from build123d import *

# Parameters (mm, degrees)
F0_R     = 19.05
F0_R_2   = 6.35
F1_DEPTH = 50.8
F3_DEPTH = 12.7


with BuildPart() as f1:
    # F0 (on Front) → F1 (new body, symmetric)
    with BuildSketch(Plane.XZ):
        Circle(F0_R)
        Circle(F0_R_2, mode=Mode.SUBTRACT)
    extrude(amount=F1_DEPTH, both=True)

    # F2 (on face) → F3 (join)
    with BuildSketch(Plane.XZ.offset(50.8)):
        with BuildLine():
            Line((-19.05, 50.8), (-19.05, 0))
            ThreePointArc((-19.05, 0), (0, 19.05), (19.05, 0))
            Line((19.05, 0), (19.05, 50.8))
            ThreePointArc((19.05, 50.8), (0, 31.75), (-19.05, 50.8))
        make_face()
        with BuildLine():
            ThreePointArc((19.05, 50.8), (0, 69.85), (-19.05, 50.8))
            Line((-19.05, 50.8), (-6.35, 50.8))
            ThreePointArc((-6.35, 50.8), (0, 57.15), (6.35, 50.8))
            Line((6.35, 50.8), (19.05, 50.8))
        make_face()
        with BuildLine():
            Line((-6.35, 50.8), (-19.05, 50.8))
            ThreePointArc((-19.05, 50.8), (0, 31.75), (19.05, 50.8))
            Line((19.05, 50.8), (6.35, 50.8))
            ThreePointArc((6.35, 50.8), (0, 44.45), (-6.35, 50.8))
        make_face()
    extrude(amount=-F3_DEPTH)

    # F4: F1 across plane


with BuildPart() as f1_1:
    add(f1.part)
    add(f1.part.mirror(Plane.XZ))


solid = f1_1.part
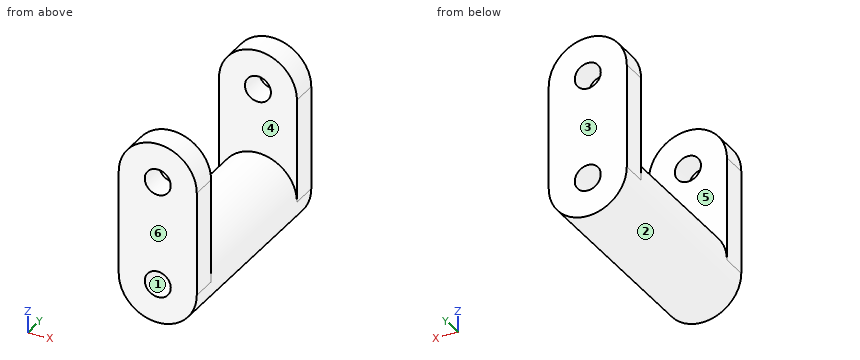
For this review, take the finished solid that the model builds, in its own axes (mm). Face numbers are marked on the shaded views. A direction names the side the tool comes from. Round coordinates to 2 decimals unless told otherwise and drop trailing zeros. Order: outer loops, then holes, each group sorted by start corner. A loop starts at its lowest first (then second) coordinate and runs counter-clockwise, first axis right, second up. Notation, with made-up numbers: M -26.5,-30.5 L -12.5,-30.5 A19 ccw -12.5,3.5 Z; hole C -29,-9.5 d5. An arc over 180 degrees is marked long. Write each question's results on one line, items separated by ' | '. Start each with the question number.
1. Draft analysis for pull direction Y (two halves, no side actions). For the marked faces 3, 4, 5 and 6, state which applies: pulls with the +Y half, pulls with the -Y half, needs draft (parallel to the pull), parting line crosses it, or undercut.
2. Add section C-C (y = -27.5). State the section outline as (x, z) points.
3. Tool access review of the marked faces 1 and 2: name each direction out of +Z, -Z, +X, -X, +Y, -Y from which nothing blocks a thin tool from reaching the whole face with its end or side.
4. Add section B-B (z = 24.5). State the section outline as (x, y) points, then the cut area to 3 significant figures.
5. Add section D-D (z = 46). State the section outline as (x, y) points, then the cut area to 3 significant figures.
6. Clearance check with flat-ended pins moving along their axes: pin 1 Ø8 at (x, y) = (9, 35.5) entering from -Z; pin 2 Ø8 at (y, z) = (22, 8) entering from -X; pin 3 Ø4 at (x, y) = (9, -4) entering from -Z; pin 4 Ø6 at (y, z) = (33, 49) entering from -X. State where each tip first meets the part, or that it passes through.
7. To check wall thickness, follow L1, parallel to Z at x = 0, y = -45.25; L2, parallel to Y at x = -14, z = 52.5; L3, parallel to X at y = 38, z = -0.5. State the ranges of each line that lie inside material, in increasing order. Write a range as [from, to].
8. Add section A-A (x = 0). State the section outline as (y, z) points, then the cut area to 3 significant figures.
Output values:
1) face 3: pulls with the +Y half | face 4: undercut | face 5: undercut | face 6: pulls with the -Y half
2) outline: C 0,0 d38.1; hole C 0,0 d12.7
3) face 1: +Y, -Y | face 2: none
4) outline: M -19.05,-50.8 L 19.05,-50.8 L 19.05,-38.1 L -19.05,-38.1 Z; M -19.05,38.1 L 19.05,38.1 L 19.05,50.8 L -19.05,50.8 Z | area: 968 mm^2
5) outline: M -19.05,-50.8 L -4.16,-50.8 L -4.16,-38.1 L -19.05,-38.1 Z; M -19.05,38.1 L -4.16,38.1 L -4.16,50.8 L -19.05,50.8 Z; M 4.16,-50.8 L 19.05,-50.8 L 19.05,-38.1 L 4.16,-38.1 Z; M 4.16,38.1 L 19.05,38.1 L 19.05,50.8 L 4.16,50.8 Z | area: 757 mm^2
6) pin 1: z = -18.38 | pin 2: x = -18.63 | pin 3: z = -17.72 | pin 4: through
7) L1: [-19.05, -6.35], [6.35, 44.45], [57.15, 69.85] | L2: [-50.8, -38.1], [38.1, 50.8] | L3: [-19.04, -6.33], [6.33, 19.04]
8) outline: M -50.8,-19.05 L 50.8,-19.05 L 50.8,-6.35 L -50.8,-6.35 Z; M -50.8,6.35 L 50.8,6.35 L 50.8,44.45 L 38.1,44.45 L 38.1,19.05 L -38.1,19.05 L -38.1,44.45 L -50.8,44.45 Z; M -50.8,57.15 L -38.1,57.15 L -38.1,69.85 L -50.8,69.85 Z; M 38.1,57.15 L 50.8,57.15 L 50.8,69.85 L 38.1,69.85 Z | area: 3,550 mm^2
